Geometry check sheet. Reference: the model listing, model coordinates, mm. A direction names the side the tool comes from. Round coordinates to 2 decimals unless told otherwise and drop trailing zeros. Write each loop counter-clockwise with the first axis right and the second up, starting at its lowest first coordinate (ties: lowest second). Pieces come first, ordered by that corner, then holes. Notation, with made-up numbers: (7, -33.75) - (12, -33.75) arc R14 ccw to (12, -14.75) - close; hole circle Ø2 at (47, -31). An arc over 180 degrees is marked (long way). Return JSON: item names as keys, results as strings.
```python
from build123d import *

# Parameters (mm, degrees)
SKETCH1_W               = 279.4
SKETCH1_H               = 152.4
BOSS_EXTRUDE1_DEPTH     = 12.7
SKETCH2_W               = 25.4
SKETCH2_H               = 12.7
BOSS_EXTRUDE2_DEPTH     = 12.7
LPATTERN1_COUNT         = 5
LPATTERN1_PITCH         = 50.8
MIRROR1_COPY_1_SKETCH_W = 25.4
MIRROR1_COPY_1_SKETCH_H = 12.7
MIRROR1_COPY_1_DEPTH    = 12.7
MIRROR1_COPY_2_SKETCH_W = 25.4
MIRROR1_COPY_2_SKETCH_H = 12.7
MIRROR1_COPY_2_DEPTH    = 12.7
MIRROR1_COPY_3_SKETCH_W = 25.4
MIRROR1_COPY_3_SKETCH_H = 12.7
MIRROR1_COPY_3_DEPTH    = 12.7
MIRROR1_COPY_4_SKETCH_W = 25.4
MIRROR1_COPY_4_SKETCH_H = 12.7
MIRROR1_COPY_4_DEPTH    = 12.7
SKETCH3_W               = 12.7
SKETCH3_H               = 25.4
BOSS_EXTRUDE3_DEPTH     = 12.7
LPATTERN2_COUNT         = 3
LPATTERN2_PITCH         = 50.8
SKETCH4_W               = 25.4
SKETCH4_H               = 12.7
CUT_EXTRUDE1_DEPTH      = 13.7
LPATTERN3_COUNT         = 2
LPATTERN3_PITCH         = 228.6
SKETCH5_W               = 25.4
SKETCH5_H               = 12.7
CUT_EXTRUDE2_DEPTH      = 13.7
LPATTERN4_COUNT         = 2
LPATTERN4_PITCH         = 228.6
SKETCH6_R               = 2.1
CUT_EXTRUDE3_DEPTH      = 13.7


with BuildPart() as part:
    # Sketch1 → Boss-Extrude1 (new body)
    with BuildSketch(Plane.XY):
        Rectangle(SKETCH1_W, SKETCH1_H)
    extrude(amount=BOSS_EXTRUDE1_DEPTH)

    # Sketch2 → Boss-Extrude2 (add)
    with BuildSketch(Plane.XZ.offset(76.2)):
        with Locations((-101.6, 6.35)):
            Rectangle(SKETCH2_W, SKETCH2_H)
    boss_extrude2 = extrude(amount=BOSS_EXTRUDE2_DEPTH)

    # LPattern1: Boss-Extrude2 ×5
    with Locations(*[(i * LPATTERN1_PITCH, 0, 0) for i in range(1, LPATTERN1_COUNT)]):
        add(boss_extrude2)

    # Mirror1: Boss-Extrude2 across plane
    add(boss_extrude2.mirror(Plane.ZX))

    # Mirror1 copy 1 sketch → Mirror1 copy 1 (add)
    with BuildSketch(Plane(origin=(50.8, 76.2, 0), x_dir=(1, 0, 0), z_dir=(0, 1, 0))):
        with Locations((-101.6, -6.35)):
            Rectangle(MIRROR1_COPY_1_SKETCH_W, MIRROR1_COPY_1_SKETCH_H)
    extrude(amount=MIRROR1_COPY_1_DEPTH)

    # Mirror1 copy 2 sketch → Mirror1 copy 2 (add)
    with BuildSketch(Plane(origin=(101.6, 76.2, 0), x_dir=(1, 0, 0), z_dir=(0, 1, 0))):
        with Locations((-101.6, -6.35)):
            Rectangle(MIRROR1_COPY_2_SKETCH_W, MIRROR1_COPY_2_SKETCH_H)
    extrude(amount=MIRROR1_COPY_2_DEPTH)

    # Mirror1 copy 3 sketch → Mirror1 copy 3 (add)
    with BuildSketch(Plane(origin=(152.4, 76.2, 0), x_dir=(1, 0, 0), z_dir=(0, 1, 0))):
        with Locations((-101.6, -6.35)):
            Rectangle(MIRROR1_COPY_3_SKETCH_W, MIRROR1_COPY_3_SKETCH_H)
    extrude(amount=MIRROR1_COPY_3_DEPTH)

    # Mirror1 copy 4 sketch → Mirror1 copy 4 (add)
    with BuildSketch(Plane(origin=(203.2, 76.2, 0), x_dir=(1, 0, 0), z_dir=(0, 1, 0))):
        with Locations((-101.6, -6.35)):
            Rectangle(MIRROR1_COPY_4_SKETCH_W, MIRROR1_COPY_4_SKETCH_H)
    extrude(amount=MIRROR1_COPY_4_DEPTH)

    # Sketch3 → Boss-Extrude3 (add)
    with BuildSketch(Plane.ZY.offset(139.7)):
        with Locations((6.35, 63.5)):
            Rectangle(SKETCH3_W, SKETCH3_H)
    boss_extrude3 = extrude(amount=BOSS_EXTRUDE3_DEPTH)

    # LPattern2: Boss-Extrude3 ×3
    with Locations(*[(0, -i * LPATTERN2_PITCH, 0) for i in range(1, LPATTERN2_COUNT)]):
        add(boss_extrude3)

    # Sketch4 → Cut-Extrude1 (cut, through all)
    with BuildSketch(Plane(origin=(0, 0, 0), x_dir=(-1, 0, 0), z_dir=(0, 0, -1))):
        with Locations((-127, 19.05)):
            Rectangle(SKETCH4_W, SKETCH4_H)
    cut_extrude1 = extrude(amount=-CUT_EXTRUDE1_DEPTH, mode=Mode.SUBTRACT)

    # LPattern3: Cut-Extrude1 ×2
    with Locations(*[(-i * LPATTERN3_PITCH, 0, 0) for i in range(1, LPATTERN3_COUNT)]):
        add(cut_extrude1, mode=Mode.SUBTRACT)

    # Sketch5 → Cut-Extrude2 (cut, through all)
    with BuildSketch(Plane.XY.offset(12.7)):
        with Locations((-101.6, 41.275)):
            Rectangle(SKETCH5_W, SKETCH5_H)
    cut_extrude2 = extrude(amount=-CUT_EXTRUDE2_DEPTH, mode=Mode.SUBTRACT)

    # LPattern4: Cut-Extrude2 ×2
    with Locations(*[(i * LPATTERN4_PITCH, 0, 0) for i in range(1, LPATTERN4_COUNT)]):
        add(cut_extrude2, mode=Mode.SUBTRACT)

    # Sketch6 → Cut-Extrude3 (cut, through all)
    with BuildSketch(Plane(origin=(0, 0, 0), x_dir=(-1, 0, 0), z_dir=(0, 0, -1))):
        with Locations((-81.986081859, 12)):
            Circle(SKETCH6_R)
        with Locations((-16.378881859, 12)):
            Circle(SKETCH6_R)
        with Locations((63.020004141, 13.50877)):
            Circle(SKETCH6_R)
        with Locations((29.870004141, 47.77)):
            Circle(SKETCH6_R)
        with Locations((63.020004141, 47.77)):
            Circle(SKETCH6_R)
        with Locations((29.870004141, 13.50877)):
            Circle(SKETCH6_R)
    extrude(amount=-CUT_EXTRUDE3_DEPTH, mode=Mode.SUBTRACT)


solid = part.part
```
(1) Access from +Z, -Z, +X, -X, +Y, -Y to the whole of each face (thin tool, end or side, straight path). Record for faces 1 (the face through (114.3, 41, 6)), 2 (the face through (25, 76.2, 6)), 3 (the face through (-88.9, 41, 6)).
Response values:
{"face 1": "+Z, -Z, +X", "face 2": "+Z, -Z, +Y", "face 3": "+Z, -Z"}
(2) Gauge pin test, flat ends, axial feed: pin 1 (3 mm diameter, centred on x = 34.5, z = 5, fed in from +Y); pin 2 (4 mm diameter, centred on y = 82.5, z = 4.5, fed in from +X); pin 3 (4 mm diameter, centred on y = -64.5, z = 7, fed in from -X); pin 4 (5.5 mm diameter, centred on x = -29.87, y = 47.77, fed in from +Z). Record the tip position at first contact, or that the pin passes through.
Response values:
{"pin 1": "stops at y = 76.2", "pin 2": "stops at x = 114.3", "pin 3": "stops at x = -139.7", "pin 4": "stops at z = 12.7"}
(3) Section check D-D, the plane y = -67.5. Enter the section's corners in (x, z), plus the area to 3 significant figures.
Response values:
{"outline": "(-139.7, 0) - (139.7, 0) - (139.7, 12.7) - (-139.7, 12.7) - close", "area": "3,550 mm^2"}
(4) Section check A-A, the plane x = -101. Enter the section's corners in (y, z) (3 decimals), plus the area to 3 significant figures.
Response values:
{"outline": "(-88.9, 0) - (12.7, 0) - (12.7, 12.7) - (-88.9, 12.7) - close; (25.4, 0) - (34.925, 0) - (34.925, 12.7) - (25.4, 12.7) - close; (47.625, 0) - (88.9, 0) - (88.9, 12.7) - (47.625, 12.7) - close", "area": "1,940 mm^2"}
(5) Release check for a two-part mould opening along X. For faces 4 (the face through (139.7, -32, 6)), 5 (the face through (-146, -50.8, 6)), 6 (the face through (-63.5, 82, 6)) record: pulls with the +X half, pulls with the -X half, needs draft (parallel to the pull), parting line crosses it, or undercut.
Response values:
{"face 4": "pulls with the +X half", "face 5": "needs draft", "face 6": "undercut"}
(6) Section check C-C, the plane z = 5.75. Give the number of separate pieces and of enclosed holes in the cut face, plus the area to 3 significant figures.
Response values:
{"separate pieces": "1", "enclosed holes": "8", "area": "45,400 mm^2"}
(7) Material ranges on line 1 along X through (y, z) = (78, 6.5); line 2 along X through (y, z) = (25, 3); line 3 along X through (y, z) = (40, 11.5), recorded low to high. Write a range as [from, to].
Response values:
{"line 1": "x = [-114.3, -88.9], [-63.5, -38.1], [-12.7, 12.7], [38.1, 63.5], [88.9, 114.3]", "line 2": "x = [-152.4, -114.3], [-88.9, 114.3]", "line 3": "x = [-139.7, -114.3], [-88.9, 114.3]"}
(8) Section check B-B, the plane x = 71.5. Enter the section's corners in (y, z).
Response values:
{"outline": "(-76.2, 0) - (76.2, 0) - (76.2, 12.7) - (-76.2, 12.7) - close"}
